For this review, take the finished solid that the model builds, in its own axes (mm). Round coordinates to 2 decimals unless told otherwise and drop trailing zeros. Order: outer loops, then holes, each group sorted by start corner. A loop starts at its lowest first (then second) coordinate and runs counter-clockwise, first axis right, second up. Notation, with made-up numbers: M 42.25,36 L 88.25,36 A25 ccw 88.25,59 Z; hole C 58.5,-0.5 d11. An arc over 180 degrees is marked long. Put each result on its own line as item: value.
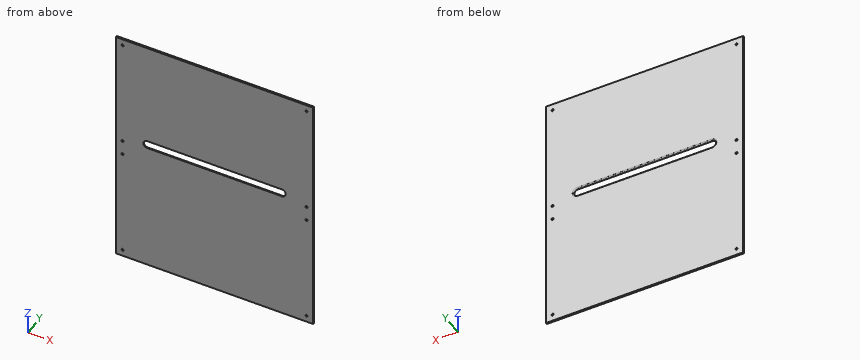
Autodesk Inventor part; units mm, degrees
ref_plane "YZ Plane" through (0, 0, 0) normal (1, 0, 0) x (0, 1, 0)
ref_plane "XZ Plane" through (0, 0, 0) normal (0, 1, 0) x (-1, 0, 0)
ref_plane "XY Plane" through (0, 0, 0) normal (0, 0, 1) x (1, 0, 0)
sketch "Sketch1" plane through (0, 0, 0) normal (0, 1, 0) x (-1, 0, 0)
  line L0 (0, 0) -> (360, 0)
  line L1 (360, 0) -> (360, -440)
  line L2 (360, -440) -> (0, -440)
  line L3 (0, -440) -> (0, 0)
  dimension "d0" = 360
  dimension "d1" = 440
extrude "Extrusion1" add sketch "Sketch1" along normal blind 3
hole "Hole1" at (-12, 3, -12) direction (0, -1, 0) diameter 4 end through all
hole "Hole2" at (-348, 3, -12) direction (0, -1, 0) diameter 4 end through all
hole "Hole3" at (-348, 3, -428) direction (0, -1, 0) diameter 4 end through all
hole "Hole4" at (-12, 3, -428) direction (0, -1, 0) diameter 4 end through all
hole "Hole5" at (-12, 3, -206.5) direction (0, -1, 0) diameter 4 end through all
hole "Hole6" at (-12, 3, -233.5) direction (0, -1, 0) diameter 4 end through all
hole "Hole7" at (-348, 3, -206.5) direction (0, -1, 0) diameter 4 end through all
hole "Hole8" at (-348, 3, -233.5) direction (0, -1, 0) diameter 4 end through all
sketch "Sketch2" plane through (0, 3, 0) normal (0, 1, 0) x (1, 0, 0)
  line L0 (-360, 440) -> (-360, 0)
  line L1 (-360, 220) -> (0, 220)
  line L2 (0, 440) -> (0, 0)
  line L3 (-310, 196) -> (-50, 196) construction
  line L4 (-303, 189) -> (-57, 189)
  line L5 (-57, 203) -> (-303, 203)
  arc A0 (-303, 203) -> (-303, 189) centre (-303, 196) ccw
  arc A1 (-57, 189) -> (-57, 203) centre (-57, 196) ccw
  point P0 (-180, 196)
extrude "Extrusion2" cut sketch "Sketch2" against normal blind 3
fillet "Fillet1" radius 2 4 edges at (-50, 3, -196) (-180, 3, -189) (-310, 3, -196) (-180, 3, -203)
properties part number "FrameTop" material "Dibond"
(1) Insertion check: pin 1 Ø2.5 at (x, z) = (-348, -233.5) entering from -Y. The pin has a flat end and moves straight along its axis. Give the tip position at first contact, or say it passes through.
A:
pin 1: passes through
(2) Add section B-B on z = -196. Give the boundary of the cut face in (x, y), then the cut area to 3 significant figures.
A:
outline: M -360,0 L -310,0 L -310,1 A2 ccw -312,3 L -360,3 Z; M -50,0 L 0,0 L 0,3 L -48,3 A2 ccw -50,1 Z
area: 298 mm2
(3) To check wall thickness, follow L1, parallel to X at y = 2.25, z = -233.5; L2, parallel to Z at x = -348, y = 1.5; L3, parallel to Z at x = -238, y = 1.45. State the ranges of each line that lie inside material, in increasing order.
A:
L1: x = -360 to -350, -346 to -14, -10 to 0
L2: z = -440 to -430, -426 to -235.5, -231.5 to -208.5, -204.5 to -14, -10 to 0
L3: z = -440 to -203.05, -188.95 to 0
(4) Add section C-C on y = 2.3. State how many separate pieces and enclosed holes the cut face has, then the cut area to 3 significant figures.
A:
separate pieces: 1
enclosed holes: 9
area: 154,000 mm2
(5) Add section A-A on x = -129.5. Give the boundary of the cut face in (y, z), then the cut area to 3 significant figures.
A:
outline: M 0,-440 L 3,-440 L 3,-205 A2 ccw 1,-203 L 0,-203 Z; M 0,-189 L 1,-189 A2 ccw 3,-187 L 3,0 L 0,0 Z
area: 1,280 mm2
